Verification items for the finished model (mm, model axes). Face numbers are marked on the shaded views. A direction names the side the tool comes from. Round coordinates to 2 decimals unless told otherwise and drop trailing zeros. Loops run counter-clockwise (first coordinate to the right, second up) from the corner with the lowest first, then second, coordinate; pieces in that order, holes last. Notation, with made-up numbers: M 15,-2 L 67,-2 A13 cw 67,14 Z; hole C 47,-12 d9. An arc over 180 degrees is marked long. One line per item, written item: value.
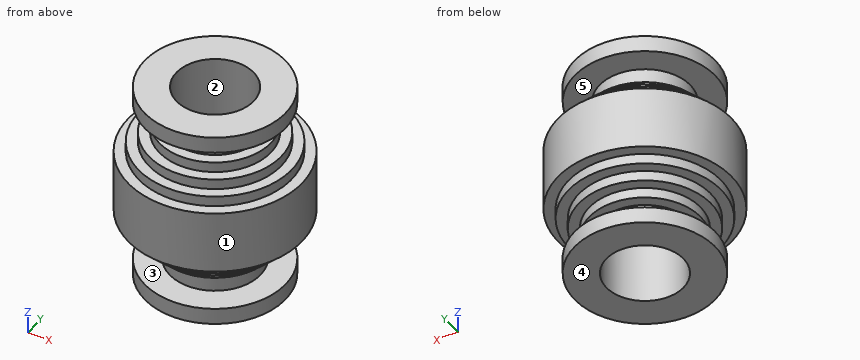
from build123d import *


with BuildPart() as part:
    # Sketch1 → Revolve1 (revolve)
    with BuildSketch(Plane(origin=(0, 0, 0), x_dir=(1, 0, 0), z_dir=(0, 1, 0)), mode=Mode.PRIVATE) as revolve1_sk:
        Polygon((4, 0), (7.3, 0), (7.3, 1.7), (4.7, 1.7), (4.7, 4), (5.775, 4), (5.775, 5.075), (6.85, 5.075), (6.85, 6.15), (7.925, 6.15), (7.925, 7.225), (9, 7.225), (9, 8.3), (9, 12.7), (9, 13.775), (7.925, 13.775), (7.925, 14.85), (6.85, 14.85), (6.85, 15.925), (5.775, 15.925), (5.775, 17), (4.7, 17), (4.7, 19.3), (7.3, 19.3), (7.3, 21), (4, 21), align=None)
    revolve(revolve1_sk.sketch.rotate(Axis((0, 0, -15), (0, 0, 1)), 180), axis=Axis((0, 0, -15), (0, 0, 1)))


solid = part.part
(1) Depth check by flat-ended pin: pin 1 Ø1 at (y, z) = (-3.5, -2.5) entering from -X; pin 2 Ø10 at (y, z) = (-7, -9) entering from +X; pin 3 Ø3 at (y, z) = (6, -14) entering from -X. Enter the tip coordinate at first touch or a pass-through.
Completed:
pin 1: stops at x = -3.62
pin 2: stops at x = 8.77
pin 3: stops at x = -7.78
(2) Tool access check on the marked faces 4 and 5. Record the directions out of +Z, -Z, +X, -X, +Y, -Y that give a thin tool (end or side, any length) a straight path to the whole face; none if there is none.
Completed:
face 4: -Z, +X, -X, +Y, -Y
face 5: none
(3) Sectioned sample at C-C on x = -5.25. Count the separate pieces of the cut face and the enclosed holes in it, and give its area (3 significant figures).
Completed:
separate pieces: 3
enclosed holes: 0
area: 185 mm^2
(4) Sectioned sample at A-A on x = 6.25. Enter the section's corners in (y, z) (3 decimals).
Completed:
outline: M -6.476,-13.775 L -4.873,-13.775 L -4.873,-14.85 L -2.804,-14.85 L -2.804,-15.925 L 2.804,-15.925 L 2.804,-14.85 L 4.873,-14.85 L 4.873,-13.775 L 6.476,-13.775 L 6.476,-7.225 L 4.873,-7.225 L 4.873,-6.15 L 2.804,-6.15 L 2.804,-5.075 L -2.804,-5.075 L -2.804,-6.15 L -4.873,-6.15 L -4.873,-7.225 L -6.476,-7.225 Z; M -3.772,-21 L 3.772,-21 L 3.772,-19.3 L -3.772,-19.3 Z; M -3.772,-1.7 L 3.772,-1.7 L 3.772,0 L -3.772,0 Z
(5) Mould release check, pull along Y, two halves, no side actions. Record for the marked faces 1, 2 and 3: +Y half, -Y half, draft (parallel to the pull), parting line (faces both ways), or undercut.
Completed:
face 1: parting line
face 2: undercut
face 3: draft
(6) Thickness scan on L1, parallel to Z at x = -4.5, y = -2.5; L2, parallel to Z at x = 6, y = -2.75 (3 decimals); L3, parallel to Y at x = 0, z = -15. Record the ranges inside material, lowest first. Write a range as from..to.
Completed:
L1: z = -21..-19.3, -17..-4, -1.7..0
L2: z = -21..-19.3, -15.925..-5.075, -1.7..0
L3: y = -6.85..-4, 4..6.85
(7) Sectioned sample at B-B on z = -11.25. Enter the section's corners in (x, y), and give its area (3 significant figures).
Completed:
outline: C 0,0 d18; hole C 0,0 d8
area: 204 mm^2
